Read the model definition and answer for the solid it produces. Units are mm, in the model's axes. Face numbers are marked on the shaded views. Give positions to 0.01 mm unless a question says otherwise; leave off trailing zeros. Write each loop counter-clockwise with the first axis right and the second up, starting at its lowest first coordinate (ties: lowest second). Pieces come first, ordered by that corner, then holes. Notation, with made-up numbers: (-40, 83) -> (7, 83) arc R9 ccw to (7, 98) -> close; hole circle Ø10 at (-1, 65.5). An arc over 180 degrees is marked (long way). Write item = value, one per line.
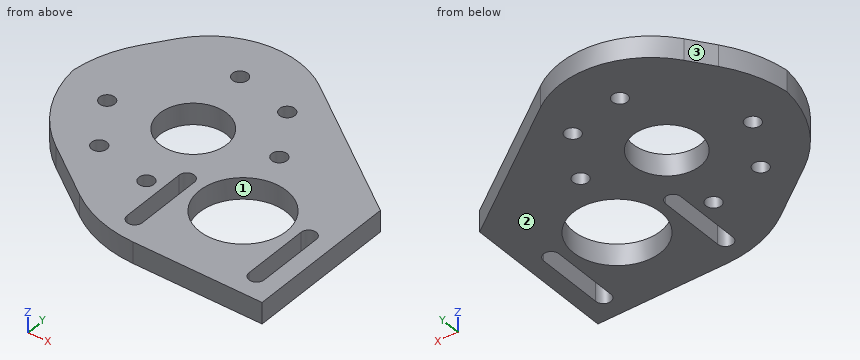
from build123d import *

# Parameters (mm, degrees)
SKETCH1_W               = 100
SKETCH1_H               = 100
BOSS_EXTRUDE1_DEPTH     = 7
SKETCH2_R               = 14.275
CUT_EXTRUDE1_DEPTH      = 142.594491418
SKETCH3_R               = 11
CUT_EXTRUDE2_DEPTH      = 10
SKETCH6_R               = 2.5
CUT_EXTRUDE3_DEPTH      = 142.594491418
CUT_EXTRUDE4_DEPTH      = 142.594491418
CUT_EXTRUDE4_DEPTH_BACK = 142.594491418
FILLET1_R               = 30
FILLET2_R               = 40


with BuildPart() as part:
    # Sketch1 → Boss-Extrude1 (new body)
    with BuildSketch(Plane.XY):
        with Locations((50, 50)):
            Rectangle(SKETCH1_W, SKETCH1_H)
    extrude(amount=BOSS_EXTRUDE1_DEPTH)

    # Sketch2 → Cut-Extrude1 (cut, through all)
    with BuildSketch(Plane.XY.offset(7)):
        with Locations((72, 28)):
            Circle(SKETCH2_R)
        with BuildLine():
            Line((54.5, 30), (54.5, 8))
            ThreePointArc((54.5, 8), (52, 5.5), (49.5, 8))
            Line((49.5, 8), (49.5, 30))
            ThreePointArc((49.5, 30), (52, 32.5), (54.5, 30))
        make_face()
        with BuildLine():
            Line((94.5, 30), (94.5, 8))
            ThreePointArc((94.5, 8), (92, 5.5), (89.5, 8))
            Line((89.5, 8), (89.5, 30))
            ThreePointArc((89.5, 30), (92, 32.5), (94.5, 30))
        make_face()
    extrude(amount=-CUT_EXTRUDE1_DEPTH, mode=Mode.SUBTRACT)

    # Sketch3 → Cut-Extrude2 (cut)
    with BuildSketch(Plane(origin=(0, 0, 0), x_dir=(-1, 0, 0), z_dir=(0, 0, -1))):
        with Locations((-40.225524413, 47.915639612)):
            Circle(SKETCH3_R)
    extrude(amount=-CUT_EXTRUDE2_DEPTH, mode=Mode.SUBTRACT)

    # Sketch6 → Cut-Extrude3 (cut, through all)
    with BuildSketch(Plane(origin=(0, 0, 0), x_dir=(-1, 0, 0), z_dir=(0, 0, -1))):
        with Locations((-15.158085821, 43.818869855)):
            Circle(SKETCH6_R)
        with Locations((-36.128754655, 72.983078204)):
            Circle(SKETCH6_R)
        with Locations((-25.397022274, 27.293430121)):
            Circle(SKETCH6_R)
        with Locations((-44.322294171, 22.848201021)):
            Circle(SKETCH6_R)
        with Locations((-55.054026552, 68.537849104)):
            Circle(SKETCH6_R)
        with Locations((-65.292963005, 52.01240937)):
            Circle(SKETCH6_R)
    extrude(amount=-CUT_EXTRUDE3_DEPTH, mode=Mode.SUBTRACT)

    # Sketch7 → Cut-Extrude4 (cut, two sides: drawn at the far end of the back side and taken through both)
    with BuildSketch(Plane(origin=(0, 0, 0), x_dir=(-1, 0, 0), z_dir=(0, 0, -1)).offset(-CUT_EXTRUDE4_DEPTH_BACK)):
        Polygon((-100, 100), (-100, 50), (-30.50895185, 100), align=None)
        Polygon((0, 100), (-30.50895185, 100), (0, 57.59801916), align=None)
        Polygon((0, 32.194859297), (-44.745090352, 0), (0, 0), align=None)
    extrude(amount=CUT_EXTRUDE4_DEPTH + CUT_EXTRUDE4_DEPTH_BACK, mode=Mode.SUBTRACT)

    # Fillet1
    fillet1_edges = [part.edges().sort_by_distance(p)[0] for p in [
        (30.50895185, 100, 3.5),
    ]]
    fillet(fillet1_edges, radius=FILLET1_R)

    # Fillet2
    # the kernel refuses this fillet: 40 mm, written as the material it takes off along each edge
    with BuildSketch(Plane(origin=(44.745090352, 0, 39.23712894), x_dir=(-0.8117201564538461, 0.5840465628753787, 0), z_dir=(0, 0, -1))) as fillet2_piece_1:
        with BuildLine():
            CenterArc((FILLET2_R * 0.322371289404, FILLET2_R), FILLET2_R, 234.264337428, 35.735662572)
            Line((-FILLET2_R * 0.261675273471, FILLET2_R * 0.188279843546), (0, 0))
            Line((0, 0), (FILLET2_R * 0.322371289404, 0))
        make_face()
    extrude(amount=71.474257881, mode=Mode.SUBTRACT)
    with BuildSketch(Plane(origin=(0, 32.194859297, -51.243453032), x_dir=(0, 1, 0), z_dir=(0, 0, 1))) as fillet2_piece_2:
        with BuildLine():
            CenterArc((FILLET2_R * 0.512434530321, -FILLET2_R), FILLET2_R, 90, 54.264337428)
            Line((-FILLET2_R * 0.299285626133, -FILLET2_R * 0.415953437125), (0, 0))
            Line((0, 0), (FILLET2_R * 0.512434530321, 0))
        make_face()
    extrude(amount=109.486906064, mode=Mode.SUBTRACT)
    with BuildSketch(Plane(origin=(0, 57.59801916, -32.23712894), x_dir=(0.5840465628753787, 0.8117201564538461, 0), z_dir=(0, 0, 1))) as fillet2_piece_3:
        with BuildLine():
            CenterArc((FILLET2_R * 0.322371289404, -FILLET2_R), FILLET2_R, 90, 35.735662572)
            Line((-FILLET2_R * 0.261675273471, -FILLET2_R * 0.188279843546), (0, 0))
            Line((0, 0), (FILLET2_R * 0.322371289404, 0))
        make_face()
    extrude(amount=71.474257881, mode=Mode.SUBTRACT)


solid = part.part
(1) For a pull along X with two mould halves and no side action, classify the marked faces 1, 2 and 3 as released by +X, released by -X, zero draft, split by the parting line, or undercut.
Checks:
face_1 = undercut
face_2 = zero draft
face_3 = released by -X
(2) The part is cut by section A-A on y = 40. Determine the outline of the cut face in (x, z).
Checks:
outline = (2.07, 0) -> (32.59, 0) -> (32.59, 7) -> (2.07, 7) -> close; (47.86, 0) -> (64.27, 0) -> (64.27, 7) -> (47.86, 7) -> close; (79.73, 0) -> (100, 0) -> (100, 7) -> (79.73, 7) -> close
(3) Given P1, Ø4, axis at y = 42, z = 3, coming from the -X side; P2, Ø4, axis at x = 44.32, y = 22.85, coming from the +Z side; P3, Ø4, axis at x = 53.5, z = 5.5, coming from the -Y side; P4, Ø2, axis at y = 22, z = 2.5, coming from the -X side, each flat-ended and moving along its own axis, determine where each tip first touches the part or whether it passes through.
Checks:
P1 = 0.96
P2 = through
P3 = 0.06
P4 = 13.2
(4) Consider L1, parallel to X at y = 8, z = 4.75; L2, parallel to X at y = 50, z = 3; L3, parallel to X at y = 31.5, z = 3.5. Determine where each line is inside the solid, lowest interval first.
Checks:
L1 = 33.63 to 49.5, 54.5 to 89.5, 94.5 to 100
L2 = 0.35 to 29.42, 51.03 to 63.81, 66.78 to 100
L3 = 6.08 to 50, 54 to 58.16, 85.84 to 90, 94 to 100
(5) The part is cut by section B-B on x = 92. Determine the outline of the cut face in (y, z).
Checks:
outline = (0, 0) -> (5.5, 0) -> (5.5, 7) -> (0, 7) -> close; (32.5, 0) -> (55.76, 0) -> (55.76, 7) -> (32.5, 7) -> close
(6) The part is cut by section D-D on x = 43. Determine the outline of the cut face in (y, z).
Checks:
outline = (2.78, 0) -> (20.73, 0) -> (20.73, 7) -> (2.78, 7) -> close; (24.97, 0) -> (37.27, 0) -> (37.27, 7) -> (24.97, 7) -> close; (58.56, 0) -> (87.59, 0) -> (87.59, 7) -> (58.56, 7) -> close
(7) The part is cut by section C-C on z = 3. Count the separate pieces of the cut face and the enclosed holes in it, plus the area to 3 significant figures.
Checks:
separate_pieces = 1
enclosed_holes = 10
area = 5,210 mm²
